The model under review builds one solid part; all positions refer to its coordinate system, in mm. Round coordinates to 2 decimals unless told otherwise and drop trailing zeros. Order: outer loops, then holes, each group sorted by start corner. A loop starts at its lowest first (then second) coordinate and runs counter-clockwise, first axis right, second up.
```python
from build123d import *

# Parameters (mm, degrees)
F0_R          = 25
F1_DEPTH      = 150
F0_R_2        = 55.1997583715
F2_DEPTH      = 50
F4_DEPTH      = 250.001
F8_DEPTH      = 60
F10_R         = 40
F11_DEPTH     = 257
F12_T1_DEPTH  = 1255
F12_T3_DEPTH  = 2500
F12_T5_DEPTH  = 603.5533905933
F12_T7_DEPTH  = 556.1937137964
F12_T9_DEPTH  = 595.9370668734
F12_T14_DEPTH = 330
F12_S15_R     = 50
F12_T16_DEPTH = 170
F12_T20_DEPTH = 330
F12_S21_R     = 50
F12_T22_DEPTH = 170
F12_T26_DEPTH = 330
F12_S27_R     = 50
F12_T28_DEPTH = 170
F12_T32_DEPTH = 330
F12_S33_R     = 50
F12_T34_DEPTH = 170
F12_T36_ANGLE = 8.4091330213
F12_T38_ANGLE = 8.4091330213


# Not quite as in the source:
# - a fillet or chamfer that OpenCascade refuses, or shapes differently, is made with other operations: its cross-section is extruded or revolved along the edge and cut away or added


with BuildPart() as f1:
    # F0 (on Front) → F1 (new body)
    with BuildSketch(Plane.XZ):
        with BuildLine():
            Line((250, 824.2658257814), (0, 1074.2658257814))
            Line((0, 1074.2658257814), (0, -1175.7341742186))
            Line((0, -1175.7341742186), (80, -1175.7341742186))
            Line((80, -1175.7341742186), (172.4239571783, -977.530358429))
            Line((172.4239571783, -977.530358429), (228.4980691431, -598.2156102055))
            ThreePointArc((228.4980691431, -598.2156102055), (244.6172738506, -452.3695412242), (250, -305.7341742186))
            Line((250, -305.7341742186), (250, 824.2658257814))
        make_face()
        with Locations((80, -675.7341742186)):
            Circle(F0_R, mode=Mode.SUBTRACT)
    extrude(amount=F1_DEPTH)

    # F0 (on Front) → F2 (join)
    with BuildSketch(Plane.XZ):
        Polygon((0, 1454.2658257814), (0, 1074.2658257814), (250, 824.2658257814), (250, 1204.2658257814), align=None)
        with Locations((100, 1244.2658257814)):
            Circle(F0_R_2, mode=Mode.SUBTRACT)
    extrude(amount=F2_DEPTH)

    # F3 (on face) → F4 (cut, through all)
    with BuildSketch(Plane(origin=(0, 0, 0), x_dir=(0, -1, 0), z_dir=(-1, 0, 0))):
        Polygon((10, -1175.7341742186), (10, -305.7341742186), (0, -305.7341742186), (0, -598.2156102055), (0, -977.530358429), (0, -1175.7341742186), align=None)
    extrude(amount=-F4_DEPTH, mode=Mode.SUBTRACT)

    # F5: F1 across plane


with BuildPart() as f1_1:
    add(f1.part)
    add(f1.part.mirror(Plane.XZ))

    # F7 (on offset) → F8 (cut, symmetric)
    with BuildSketch(Plane(origin=(0, 0, 0), x_dir=(-1, 0, 0), z_dir=(0, 1, 0))):
        with BuildLine():
            Line((-228.4980691431, -598.2156102055), (-187.4724905077, -875.7341742186))
            ThreePointArc((-187.4724905077, -875.7341742186), (-154.7929091893, -655.7842074431), (-244.6172738506, -452.3695412242))
            Line((-244.6172738506, -452.3695412242), (-228.4980691431, -598.2156102055))
        make_face()
        Polygon((-289.7645564147, -893.9040561501), (-187.4724905077, -875.7341742186), (-228.4980691431, -598.2156102055), (-244.6172738506, -452.3695412242), (-337.4301303856, -462.6274072361), align=None)
    extrude(amount=F8_DEPTH, both=True, mode=Mode.SUBTRACT)

    # F10 (on face) → F11 (cut)
    with BuildSketch(Plane(origin=(-313.6375788675, 0, -1085.0784920755), x_dir=(0.9606739331, 0, -0.2776789409), z_dir=(-0.2776789409, 0, -0.9606739331))):
        with Locations((364.9035775946, 0)):
            Circle(F10_R)
    extrude(amount=-F11_DEPTH, mode=Mode.SUBTRACT)

    # F12: fillet of radius 50 on 14 edges, made by hand

    # F12_s2 → F12_t1 (cut)
    with BuildSketch(Plane.XY.offset(-305.7341742186)):
        with BuildLine():
            ThreePointArc((250, -100), (235.3553390593, -135.3553390593), (200, -150))
            Line((200, -150), (250, -150))
            Line((250, -150), (250, -100))
        make_face()
        with BuildLine():
            ThreePointArc((250, 100), (235.3553390593, 135.3553390593), (200, 150))
            Line((200, 150), (250, 150))
            Line((250, 150), (250, 100))
        make_face()
    extrude(amount=F12_T1_DEPTH, mode=Mode.SUBTRACT)

    # F12_s4 → F12_t3 (cut)
    with BuildSketch(Plane.XY.offset(-1300.7341742186)):
        with BuildLine():
            ThreePointArc((50, -150), (14.6446609407, -135.3553390593), (0, -100))
            Line((0, -100), (0, -150))
            Line((0, -150), (50, -150))
        make_face()
        with BuildLine():
            ThreePointArc((50, 150), (14.6446609407, 135.3553390593), (0, 100))
            Line((0, 100), (0, 150))
            Line((0, 150), (50, 150))
        make_face()
    extrude(amount=F12_T3_DEPTH, mode=Mode.SUBTRACT)

    # F12_s6 → F12_t5 (cut)
    with BuildSketch(Plane(origin=(-198.7445652424, 0, 198.7445652424), x_dir=(0, 1, 0), z_dir=(-0.7071067812, 0, 0.7071067812))):
        with BuildLine():
            ThreePointArc((-150, -709.620650207), (-135.3553390593, -744.9759892663), (-100, -759.620650207))
            Line((-100, -759.620650207), (-150, -759.620650207))
            Line((-150, -759.620650207), (-150, -709.620650207))
        make_face()
        with BuildLine():
            ThreePointArc((100, -759.620650207), (135.3553390593, -744.9759892663), (150, -709.620650207))
            Line((150, -709.620650207), (150, -759.620650207))
            Line((150, -759.620650207), (100, -759.620650207))
        make_face()
    extrude(amount=F12_T5_DEPTH, mode=Mode.SUBTRACT)

    # F12_s8 → F12_t7 (cut)
    with BuildSketch(Plane(origin=(-488.8711024777, 0, -1048.3874625005), x_dir=(0, 1, 0), z_dir=(0.4226182617, 0, 0.906307787))):
        with BuildLine():
            ThreePointArc((-150, -519.3913559403), (-135.3553390593, -554.7466949997), (-100, -569.3913559403))
            Line((-100, -569.3913559403), (-150, -569.3913559403))
            Line((-150, -569.3913559403), (-150, -519.3913559403))
        make_face()
        with BuildLine():
            ThreePointArc((150, -519.3913559403), (135.3553390593, -554.7466949997), (100, -569.3913559403))
            Line((100, -569.3913559403), (150, -569.3913559403))
            Line((150, -569.3913559403), (150, -519.3913559403))
        make_face()
    extrude(amount=F12_T7_DEPTH, mode=Mode.SUBTRACT)

    # F12_s10 → F12_t9 (cut)
    with BuildSketch(Plane(origin=(-168.8064738845, 0, -1141.8956608733), x_dir=(0, 1, 0), z_dir=(0.146240718, 0, 0.9892490346))):
        with BuildLine():
            ThreePointArc((-150, -263.5249746526), (-135.3553390593, -298.8803137119), (-100, -313.5249746526))
            Line((-100, -313.5249746526), (-150, -313.5249746526))
            Line((-150, -313.5249746526), (-150, -263.5249746526))
        make_face()
        with BuildLine():
            ThreePointArc((150, -263.5249746526), (135.3553390593, -298.8803137119), (100, -313.5249746526))
            Line((100, -313.5249746526), (150, -313.5249746526))
            Line((150, -313.5249746526), (150, -263.5249746526))
        make_face()
    extrude(amount=F12_T9_DEPTH, mode=Mode.SUBTRACT)


with BuildPart() as f12_tool12:
    # F12_s13 → F12_t14 (new body)
    with BuildSketch(Plane.YZ.offset(-125)):
        with BuildLine():
            ThreePointArc((-150, -1125.7341742186), (-135.3553390593, -1161.0895132779), (-100, -1175.7341742186))
            Line((-100, -1175.7341742186), (-150, -1175.7341742186))
            Line((-150, -1175.7341742186), (-150, -1125.7341742186))
        make_face()
    extrude(amount=F12_T14_DEPTH)

    # F12_s15 → F12_t16 (cut, symmetric)
    with BuildSketch(Plane(origin=(-433.606336546, 0, -929.8717894996), x_dir=(0, 1, 0), z_dir=(-0.4226182617, 0, -0.906307787))):
        with Locations((-100, 519.3913559403)):
            Circle(F12_S15_R)
    extrude(amount=F12_T16_DEPTH, both=True, mode=Mode.SUBTRACT)


with BuildPart() as f1_2:
    add(f1_1.part)

    # F12_t11: cut F12_tool12
    add(f12_tool12.part, mode=Mode.SUBTRACT)


with BuildPart() as f12_tool18:
    # F12_s19 → F12_t20 (new body)
    with BuildSketch(Plane.YZ.offset(-125)):
        with BuildLine():
            ThreePointArc((-150, -1125.7341742186), (-135.3553390593, -1161.0895132779), (-100, -1175.7341742186))
            Line((-100, -1175.7341742186), (-150, -1175.7341742186))
            Line((-150, -1175.7341742186), (-150, -1125.7341742186))
        make_face()
    extrude(amount=F12_T20_DEPTH)

    # F12_s21 → F12_t22 (cut, symmetric)
    with BuildSketch(Plane.XY.offset(-1150.7)):
        with Locations((50, -100)):
            Circle(F12_S21_R)
    extrude(amount=F12_T22_DEPTH, both=True, mode=Mode.SUBTRACT)


with BuildPart() as f1_3:
    add(f1_2.part)

    # F12_t17: cut F12_tool18
    add(f12_tool18.part, mode=Mode.SUBTRACT)


with BuildPart() as f12_tool24:
    # F12_s25 → F12_t26 (new body)
    with BuildSketch(Plane.YZ.offset(-125)):
        with BuildLine():
            ThreePointArc((150, -1125.7341742186), (135.3553390593, -1161.0895132779), (100, -1175.7341742186))
            Line((100, -1175.7341742186), (150, -1175.7341742186))
            Line((150, -1175.7341742186), (150, -1125.7341742186))
        make_face()
    extrude(amount=F12_T26_DEPTH)

    # F12_s27 → F12_t28 (cut, symmetric)
    with BuildSketch(Plane(origin=(-433.606336546, 0, -929.8717894996), x_dir=(0, 1, 0), z_dir=(-0.4226182617, 0, -0.906307787))):
        with Locations((100, 519.3913559403)):
            Circle(F12_S27_R)
    extrude(amount=F12_T28_DEPTH, both=True, mode=Mode.SUBTRACT)


with BuildPart() as f1_4:
    add(f1_3.part)

    # F12_t23: cut F12_tool24
    add(f12_tool24.part, mode=Mode.SUBTRACT)


with BuildPart() as f12_tool30:
    # F12_s31 → F12_t32 (new body)
    with BuildSketch(Plane.YZ.offset(-125)):
        with BuildLine():
            ThreePointArc((150, -1125.7341742186), (135.3553390593, -1161.0895132779), (100, -1175.7341742186))
            Line((100, -1175.7341742186), (150, -1175.7341742186))
            Line((150, -1175.7341742186), (150, -1125.7341742186))
        make_face()
    extrude(amount=F12_T32_DEPTH)

    # F12_s33 → F12_t34 (cut, symmetric)
    with BuildSketch(Plane.XY.offset(-1150.7)):
        with Locations((50, 100)):
            Circle(F12_S33_R)
    extrude(amount=F12_T34_DEPTH, both=True, mode=Mode.SUBTRACT)


with BuildPart() as f1_5:
    add(f1_4.part)

    # F12_t29: cut F12_tool30
    add(f12_tool30.part, mode=Mode.SUBTRACT)

    # F12_s35 → F12_t36 (revolve, cut)
    with BuildSketch(Plane(origin=(-81.6562093461, 0, -552.3654928034), x_dir=(0, 1, 0), z_dir=(-0.146240718, 0, -0.9892490346))):
        with BuildLine():
            ThreePointArc((-100, 313.5249746526), (-135.3553390593, 298.8803137119), (-150, 263.5249746526))
            Line((-150, 263.5249746526), (-150, 313.5249746526))
            Line((-150, 313.5249746526), (-100, 313.5249746526))
        make_face()
    revolve(axis=Axis((-1749.9999999999, -150, -305.7341742186), (0, -1, 0)), revolution_arc=F12_T36_ANGLE, mode=Mode.SUBTRACT)

    # F12_s37 → F12_t38 (revolve, cut)
    with BuildSketch(Plane(origin=(-81.6562093461, 0, -552.3654928034), x_dir=(0, 1, 0), z_dir=(-0.146240718, 0, -0.9892490346))):
        with BuildLine():
            ThreePointArc((150, 263.5249746526), (135.3553390593, 298.8803137119), (100, 313.5249746526))
            Line((100, 313.5249746526), (150, 313.5249746526))
            Line((150, 313.5249746526), (150, 263.5249746526))
        make_face()
    revolve(axis=Axis((-1749.9999999999, 150, -305.7341742186), (0, -1, 0)), revolution_arc=F12_T38_ANGLE, mode=Mode.SUBTRACT)


solid = f1_5.part
```
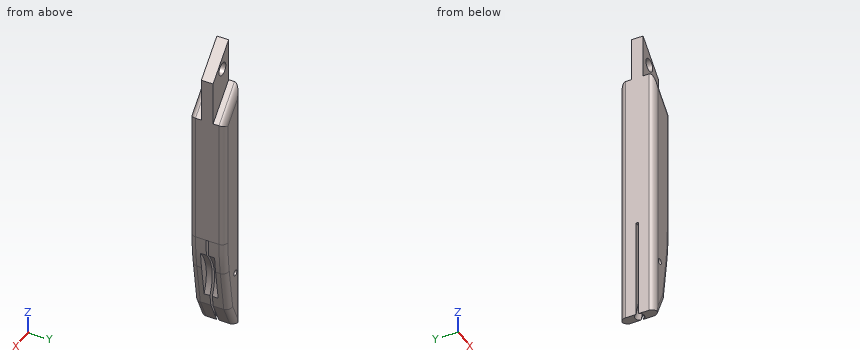
(1) Consider section A-A (z = 148.5). Write out the cut boundary in (x, y).
Data:
outline: (0, -100) arc R50 ccw to (50, -150) - (200, -150) arc R50 ccw to (250, -100) - (250, 100) arc R50 ccw to (200, 150) - (50, 150) arc R50 ccw to (0, 100) - close
(2) Insertion check: pin 1 (1.5 mm diameter, centred on x = 92.5, y = -94, fed in from -Z); pin 2 (1.5 mm diameter, centred on y = -117.5, z = -587.5, fed in from +X); pin 3 (6 mm diameter, centred on x = 110, y = 32.5, fed in from +Z). Each pin has a flat end and moves straight along its axis. Give the tip position at first contact, or say it passes through.
Data:
pin 1: stops at z = -1150.54
pin 2: stops at x = 227.15
pin 3: stops at z = 1347.27
(3) Consider section B-B (z = 1138). Write out the cut boundary in (x, y), and give its area (3 significant figures).
Data:
outline: (0, -50) - (250, -50) - (250, 50) - (0, 50) - close
area: 25,000 mm2
(4) To check wall thickness, follow probe 1 along Y at (x, z) = (188.5, -522.5); probe 2 along Z at (x, y) = (98.5, 66.5); probe 3 along Y at (x, z) = (143.5, -918). State the ranges of each line that lie inside material, in increasing order.
Data:
probe 1: y = -150 to -10, 10 to 150
probe 2: z = -1136.06 to -692.55, -658.92 to 975.77
probe 3: y = -148.37 to -10, 10 to 148.37
